```python
from build123d import *

# Parameters (mm, degrees)
F1_DEPTH     = 24
F2_R         = 1.7
F3_DEPTH     = 2
F4_R         = 5.5
F5_T1_DEPTH  = 2
F6_W         = 2
F6_H         = 6.35
F7_DEPTH     = 20
F8_R         = 5
F9_T4_DEPTH  = 2
F9_T9_DEPTH  = 12.7751879692
F9_T15_DEPTH = 2
F9_T20_DEPTH = 2
F9_T25_DEPTH = 2
F9_T30_DEPTH = 12.7751879692
F10_R        = 2.2
F11_DEPTH    = 8
F10_R_2      = 3.6
F12_DEPTH    = 4
F13_R        = 1
F14_DEPTH    = 3.6
F15_R        = 2


# Not quite as in the source:
# - a fillet or chamfer that OpenCascade refuses, or shapes differently, is made with other operations: its cross-section is extruded or revolved along the edge and cut away or added


with BuildPart() as f1:
    # F0 (on Front) → F1 (new body, symmetric)
    with BuildSketch(Plane.XZ):
        Polygon((-23.3, 12.3), (-23.3, 0), (0, 0), (23.3, 0), (23.3, 12.3), (21.3, 12.3), (17, 8), (0, 8), (-17, 8), (-21.3, 12.3), align=None)
    extrude(amount=F1_DEPTH, both=True)

    # F2 (on face) → F3 (join)
    with BuildSketch(Plane.XZ.offset(24)):
        Polygon((-23.3, 18.65), (-23.3, 12.3), (-21.3, 12.3), (-17, 8), (-10.3, 8), (-10.3, 18.65), align=None)
        with Locations((-15.5, 13.65)):
            Circle(F2_R, mode=Mode.SUBTRACT)
        Polygon((21.3, 12.3), (23.3, 12.3), (23.3, 18.65), (10.3, 18.65), (10.3, 8), (17, 8), align=None)
        with Locations((15.5, 13.65)):
            Circle(F2_R, mode=Mode.SUBTRACT)
        Polygon((-21.3, 12.3), (-23.3, 12.3), (-23.3, 0), (23.3, 0), (23.3, 12.3), (21.3, 12.3), (17, 8), (10.3, 8), (-10.3, 8), (-17, 8), align=None)
    extrude(amount=F3_DEPTH)

    # F4
    f4_edges = [f1.edges().sort_by_distance(p)[0] for p in [
        (-10.3, -25, 18.65),
        (10.3, -25, 18.65),
    ]]
    fillet(f4_edges, radius=F4_R)

    # F5: fillet of radius 10 on 2 edges, made by hand

    # F5_s2 → F5_t1 (join)
    with BuildSketch(Plane.XZ.offset(24)):
        with BuildLine():
            ThreePointArc((-1.0783322956, 8), (-6.9396323825, 9.8978298407), (-10.5761824275, 14.8709677419))
            Line((-10.5761824275, 14.8709677419), (-11.5259674406, 14.5580645161))
            ThreePointArc((-11.5259674406, 14.5580645161), (-11.3, 13.15), (-11.3, 8))
            Line((-11.3, 8), (-10.3, 7))
            Line((-10.3, 7), (-1.0783322956, 7))
            Line((-1.0783322956, 7), (-1.0783322956, 8))
        make_face()
        with BuildLine():
            ThreePointArc((10.5761824275, 14.8709677419), (6.9396323825, 9.8978298407), (1.0783322956, 8))
            Line((1.0783322956, 8), (1.0783322956, 7))
            Line((1.0783322956, 7), (10.3, 7))
            Line((10.3, 7), (11.3, 8))
            ThreePointArc((11.3, 8), (11.3, 13.15), (11.5259674406, 14.5580645161))
            Line((11.5259674406, 14.5580645161), (10.5761824275, 14.8709677419))
        make_face()
    extrude(amount=F5_T1_DEPTH)

    # F6 (on face) → F7 (join)
    with BuildSketch(Plane(origin=(0, -24, 0), x_dir=(-1, 0, 0), z_dir=(0, 1, 0))):
        with Locations((-22.3, 15.475)):
            Rectangle(F6_W, F6_H)
        with Locations((22.3, 15.475)):
            Rectangle(F6_W, F6_H)
    extrude(amount=F7_DEPTH)

    # F8
    f8_edges = [f1.edges().sort_by_distance(p)[0] for p in [
        (22.3, -4, 18.65),
        (-22.3, -4, 18.65),
    ]]
    fillet(f8_edges, radius=F8_R)

    # F9: fillet of radius 5 on 2 edges, made by hand


with BuildPart() as f9_tool2:
    # F9_s3 → F9_t4 (new body)
    with BuildSketch(Plane.YZ.offset(-21.3)):
        with BuildLine():
            ThreePointArc((-4.3449624062, 15.475), (-2.5072817297, 13.1693220895), (0.3100751877, 12.3))
            Line((0.3100751877, 12.3), (0.3100751877, 11.8))
            Line((0.3100751877, 11.8), (-4, 11.8))
            Line((-4, 11.8), (-4.5, 12.3))
            ThreePointArc((-4.5, 12.3), (-4.5, 13.65), (-4.8104661656, 15.2925))
            Line((-4.8104661656, 15.2925), (-4.3449624062, 15.475))
        make_face()
    extrude(amount=-F9_T4_DEPTH)

    split(bisect_by=Plane(origin=(-4.5, 0, -4.5), x_dir=(0, 1, 0), z_dir=(0.7071067812, 0, 0.7071067812)), keep=Keep.TOP)


with BuildPart() as f1_1:
    add(f1.part)

    # F9_t1: union F9_tool2
    add(f9_tool2.part)


with BuildPart() as f9_tool7:
    # F9_s8 → F9_t9 (new body)
    with BuildSketch(Plane.YZ.offset(-10.5248120308)):
        with BuildLine():
            ThreePointArc((-4.3449624062, 15.475), (-2.5072817297, 13.1693220895), (0.3100751877, 12.3))
            Line((0.3100751877, 12.3), (0.3100751877, 11.8))
            Line((0.3100751877, 11.8), (-4, 11.8))
            Line((-4, 11.8), (-4.5, 12.3))
            ThreePointArc((-4.5, 12.3), (-4.5, 13.65), (-4.8104661656, 15.2925))
            Line((-4.8104661656, 15.2925), (-4.3449624062, 15.475))
        make_face()
    extrude(amount=-F9_T9_DEPTH)

    split(bisect_by=Plane.YZ.offset(-21.3), keep=Keep.TOP)

    split(bisect_by=Plane(origin=(-4.5, 0, -4.5), x_dir=(0, 1, 0), z_dir=(-0.7071067812, 0, -0.7071067812)), keep=Keep.TOP)


with BuildPart() as f1_2:
    add(f1_1.part)

    # F9_t6: union F9_tool7
    add(f9_tool7.part)


with BuildPart() as f9_tool13:
    # F9_s14 → F9_t15 (new body)
    with BuildSketch(Plane.YZ.offset(-21.3)):
        with BuildLine():
            ThreePointArc((-4.3449624062, 15.475), (-2.5072817297, 13.1693220895), (0.3100751877, 12.3))
            Line((0.3100751877, 12.3), (0.3100751877, 11.8))
            Line((0.3100751877, 11.8), (-4, 11.8))
            Line((-4, 11.8), (-4.5, 12.3))
            ThreePointArc((-4.5, 12.3), (-4.5, 13.65), (-4.8104661656, 15.2925))
            Line((-4.8104661656, 15.2925), (-4.3449624062, 15.475))
        make_face()
    extrude(amount=-F9_T15_DEPTH)

    split(bisect_by=Plane(origin=(-4.5, 0, -4.5), x_dir=(0, 1, 0), z_dir=(-0.7071067812, 0, -0.7071067812)), keep=Keep.TOP)


with BuildPart() as f1_3:
    add(f1_2.part)

    # F9_t12: union F9_tool13
    add(f9_tool13.part)


with BuildPart() as f9_tool18:
    # F9_s19 → F9_t20 (new body)
    with BuildSketch(Plane.YZ.offset(23.3)):
        with BuildLine():
            ThreePointArc((0.3100751877, 12.3), (-2.5072817297, 13.1693220895), (-4.3449624062, 15.475))
            Line((-4.3449624062, 15.475), (-4.8104661656, 15.2925))
            ThreePointArc((-4.8104661656, 15.2925), (-4.5, 13.65), (-4.5, 12.3))
            Line((-4.5, 12.3), (-4, 11.8))
            Line((-4, 11.8), (0.3100751877, 11.8))
            Line((0.3100751877, 11.8), (0.3100751877, 12.3))
        make_face()
    extrude(amount=-F9_T20_DEPTH)

    split(bisect_by=Plane(origin=(4.5, 0, -4.5), x_dir=(0, 1, 0), z_dir=(0.7071067812, 0, -0.7071067812)), keep=Keep.TOP)


with BuildPart() as f1_4:
    add(f1_3.part)

    # F9_t17: union F9_tool18
    add(f9_tool18.part)


with BuildPart() as f9_tool23:
    # F9_s24 → F9_t25 (new body)
    with BuildSketch(Plane.YZ.offset(23.3)):
        with BuildLine():
            ThreePointArc((0.3100751877, 12.3), (-2.5072817297, 13.1693220895), (-4.3449624062, 15.475))
            Line((-4.3449624062, 15.475), (-4.8104661656, 15.2925))
            ThreePointArc((-4.8104661656, 15.2925), (-4.5, 13.65), (-4.5, 12.3))
            Line((-4.5, 12.3), (-4, 11.8))
            Line((-4, 11.8), (0.3100751877, 11.8))
            Line((0.3100751877, 11.8), (0.3100751877, 12.3))
        make_face()
    extrude(amount=-F9_T25_DEPTH)

    split(bisect_by=Plane(origin=(4.5, 0, -4.5), x_dir=(0, 1, 0), z_dir=(-0.7071067812, 0, 0.7071067812)), keep=Keep.TOP)


with BuildPart() as f1_5:
    add(f1_4.part)

    # F9_t22: union F9_tool23
    add(f9_tool23.part)


with BuildPart() as f9_tool28:
    # F9_s29 → F9_t30 (new body)
    with BuildSketch(Plane.YZ.offset(23.3)):
        with BuildLine():
            ThreePointArc((0.3100751877, 12.3), (-2.5072817297, 13.1693220895), (-4.3449624062, 15.475))
            Line((-4.3449624062, 15.475), (-4.8104661656, 15.2925))
            ThreePointArc((-4.8104661656, 15.2925), (-4.5, 13.65), (-4.5, 12.3))
            Line((-4.5, 12.3), (-4, 11.8))
            Line((-4, 11.8), (0.3100751877, 11.8))
            Line((0.3100751877, 11.8), (0.3100751877, 12.3))
        make_face()
    extrude(amount=-F9_T30_DEPTH)

    split(bisect_by=Plane(origin=(4.5, 0, -4.5), x_dir=(0, 1, 0), z_dir=(0.7071067812, 0, -0.7071067812)), keep=Keep.TOP)

    split(bisect_by=Plane.YZ.offset(21.3), keep=Keep.BOTTOM)


with BuildPart() as f1_6:
    add(f1_5.part)

    # F9_t27: union F9_tool28
    add(f9_tool28.part)

    # F10 (on face) → F11 (cut)
    with BuildSketch(Plane.XY.offset(8)):
        with Locations((10, -6)):
            Circle(F10_R)
        with Locations((-10, -6)):
            Circle(F10_R)
    extrude(amount=-F11_DEPTH, mode=Mode.SUBTRACT)

    # F10 (on face) → F12 (cut)
    with BuildSketch(Plane.XY.offset(8)):
        with Locations((10, -6)):
            Circle(F10_R_2)
        with Locations((10, -6)):
            Circle(F10_R, mode=Mode.SUBTRACT)
        with Locations((-10, -6)):
            Circle(F10_R_2)
        with Locations((-10, -6)):
            Circle(F10_R, mode=Mode.SUBTRACT)
    extrude(amount=-F12_DEPTH, mode=Mode.SUBTRACT)

    # F13 (on face) → F14 (cut)
    with BuildSketch(Plane(origin=(0, 0, 0), x_dir=(1, 0, 0), z_dir=(0, 0, -1))):
        with Locations((6.116718427, 3.178630789)):
            Circle(F13_R)
        with Locations((6.116718427, 8.821369211)):
            Circle(F13_R)
        with Locations((11.483281573, 10.5650712782)):
            Circle(F13_R)
        with Locations((11.483281573, 1.4349287218)):
            Circle(F13_R)
        with Locations((14.8, 6)):
            Circle(F13_R)
        with Locations((-11.483281573, 10.5650712782)):
            Circle(F13_R)
        with Locations((-14.8, 6)):
            Circle(F13_R)
        with Locations((-11.483281573, 1.4349287218)):
            Circle(F13_R)
        with Locations((-6.116718427, 3.178630789)):
            Circle(F13_R)
        with Locations((-6.116718427, 8.821369211)):
            Circle(F13_R)
    extrude(amount=-F14_DEPTH, mode=Mode.SUBTRACT)

    # F15
    f15_edges = [f1_6.edges().sort_by_distance(p)[0] for p in [
        (-23.3, 24, 6.15),
        (23.3, 24, 6.15),
        (-23.3, -26, 9.325),
        (23.3, -26, 9.325),
    ]]
    fillet(f15_edges, radius=F15_R)


solid = f1_6.part
```
Can you work these out from the model? Positions are in its coordinate system, mm. A direction names the side the tool comes from. Coordinates: 2 decimals unless noted, no trailing zeros. Order: outer loops, then holes, each group sorted by start corner. A loop starts at its lowest first (then second) coordinate and runs counter-clockwise, first axis right, second up.
1. I need wall thicknesses on line 1 (Z direction, x = 15.5, y = -25.3); line 2 (Y direction, x = 10, z = 1.6); line 3 (Z direction, x = 13.5, y = 3.5). Which ranges of each line are inside material? Lowest first, please.
2. If we section it at C-C (x = -14.8): Please give me the cut outline in (y, z).
3. If we section it at D-D (z = 13.65): Please give me the cut outline in (x, y).
4. Thinking about a two-plate mould opening in Y: for faces 1 (the face through (10.484, -1.479, 1.775)), 2 (the face through (-22, 12, 12.3)), 3 (the face through (0, 24, 5)), which applies, +Y half, -Y half, draft (parallel to the pull), parting line (faces both ways), or undercut?
5. I'm going to push flat-ended pins straight in: pin 1 (10 mm diameter, centred on x = -9, y = 4.5, fed in from +Z); pin 2 (3.5 mm diameter, centred on x = 8.5, y = -6, fed in from +Z); pin 3 (1.2 mm diameter, centred on x = 14.8, y = -6, fed in from -Z); pin 4 (8 mm diameter, centred on x = -2.5, z = 13, fed in from +Y). Where does each tip first touch, or does it pass through?
6. If we section it at B-B (z = 6.5): Please give me the cut outline in (x, y).
7. If we section it at A-A (y = 6): Please give me the cut outline in (x, z).
8. For faces 4 (the face through (12, -4, 4)), 5 (the face through (-12.54, -25.01, 17.58)), 6 (the face through (-6, -3, 3.6)), 7 (the face through (19, 0, 10)), which set-ups out of +Z, -Z, +X, -X, +Y, -Y let a thin tool reach every point of the face, with its end or its side?
Entries:
1. line 1: z = 0 to 11.95, 15.35 to 18.64
1. line 2: y = -26 to -8.2, -3.8 to 24
1. line 3: z = 0 to 8
2. outline: (-26, 0) - (-7, 0) - (-7, 3.6) - (-5, 3.6) - (-5, 0) - (24, 0) - (24, 8) - (-24, 8) - (-24, 12.1) - (-26, 12.1) - close; (-26, 15.2) - (-24, 15.2) - (-24, 18.56) - (-26, 18.56) - close
3. outline: (-23.3, -24) arc R2 ccw to (-21.3, -26) - (-17.2, -26) - (-17.2, -24) - (-21.3, -24) - (-21.3, -3.11) - (-23.3, -3.11) - close; (-13.8, -26) - (-10.08, -26) - (-10.08, -24) - (-13.8, -24) - close; (10.08, -26) - (13.8, -26) - (13.8, -24) - (10.08, -24) - close; (17.2, -26) - (21.3, -26) arc R2 ccw to (23.3, -24) - (23.3, -3.11) - (21.3, -3.11) - (21.3, -24) - (17.2, -24) - close
4. face 1: undercut
4. face 2: draft
4. face 3: +Y half
5. pin 1: stops at z = 8
5. pin 2: stops at z = 4
5. pin 3: stops at z = 3.6
5. pin 4: passes through
6. outline: (-23.3, -24) arc R2 ccw to (-21.3, -26) - (21.3, -26) arc R2 ccw to (23.3, -24) - (23.3, 22) arc R2 ccw to (21.3, 24) - (-21.3, 24) arc R2 ccw to (-23.3, 22) - close; hole circle Ø7.2 at (-10, -6); hole circle Ø7.2 at (10, -6)
7. outline: (-23.3, 0) - (23.3, 0) - (23.3, 12.3) - (21.3, 12.3) - (17, 8) - (-17, 8) - (-21.3, 12.3) - (-23.3, 12.3) - close
8. face 4: +Z
8. face 5: +Z, +Y, -Y
8. face 6: -Z
8. face 7: +Z, +Y
